Can you work these out from the model? Positions are in its coordinate system, mm. A direction names the side the tool comes from. Give positions to 0.01 mm unless a question says otherwise; leave off trailing zeros. Write each loop counter-clockwise with the first axis right and the second up, starting at its lowest first coordinate (ties: lowest second). Pieces come first, ordered by that corner, then holes.
1. Suppose I cut it at A-A (y = 0). Please give me the cut outline in (x, z).
2. Suppose I cut it at C-C (x = -20.5). Please give me the cut outline in (y, z), and give its area (3 significant figures).
3. On a 3-axis mill with a long thin cutter (end or side, diameter ignored), from which of +Z, -Z, +X, -X, +Y, -Y can I reach the whole of each face in a straight line? I mean faces 1 (the cylindrical face through (-6, 0, 91)), 2 (the flat face through (5, -5, 0)), 3 (the cylindrical face through (5.723, -1.802, 8.536)). Say none if no direction works.
4. I'm going to push flat-ended pins straight in: pin 1 (4 mm diameter, centred on x = -7, z = 67, fed in from +Y); pin 2 (12 mm diameter, centred on x = -18.5, z = 29, fed in from +Y); pin 3 (10 mm diameter, centred on x = -5.5, z = 74, fed in from -Y). Where does each tip first touch, or does it pass through?
5. Suppose I cut it at D-D (z = 70.5). Please give me the cut outline in (x, y), and give its area (3 significant figures).
6. If I drill on probe 1 along Y at (x, z) = (0, 95); probe 2 along Z at (x, y) = (-4.5, 6), over which ranges is the centre line in solid material (lowest first)?
7. Thinking about a two-plate mould opening in X: for faces 4 (the cylindrical face through (-2.11, -0.34, 65.48)), 5 (the cylindrical face through (-0.35, -1.269, 34.667)), 6 (the cylindrical face through (23.09, -9.58, 49.3)), which applies, pulls with the +X half, pulls with the -X half, needs draft (parallel to the pull), parting line crosses it, or undercut?
8. Suppose I cut it at B-B (x = 0). Please give me the cut outline in (y, z), and give its area (3 significant figures).
```python
from build123d import *

# Parameters (mm, degrees)
F0_R          = 25
F1_DEPTH      = 100
F2_R          = 9.75
F3_DEPTH      = 25.001
F3_DEPTH_BACK = 25
F4_R          = 9.75
F5_DEPTH      = 25.0010001
F5_DEPTH_BACK = 25
F6_R          = 6
F7_DEPTH      = 25
F8_R          = 6
F9_DEPTH      = 25


with BuildPart() as f1:
    # F0 (on Top) → F1 (new body)
    with BuildSketch(Plane.XY):
        Circle(F0_R)
    extrude(amount=F1_DEPTH)

    # F2 (on Right) → F3 (cut, two sides)
    with BuildSketch(Plane.YZ) as f3_sk:
        with Locations((0, 25)):
            Circle(F2_R)
    extrude(amount=F3_DEPTH, mode=Mode.SUBTRACT)
    extrude(f3_sk.sketch, amount=-F3_DEPTH_BACK, mode=Mode.SUBTRACT)

    # F4 (on Front) → F5 (cut, two sides)
    with BuildSketch(Plane.XZ) as f5_sk:
        with Locations((0, 75)):
            Circle(F4_R)
    extrude(amount=-F5_DEPTH, mode=Mode.SUBTRACT)
    extrude(f5_sk.sketch, amount=F5_DEPTH_BACK, mode=Mode.SUBTRACT)

    # F6 (on face) → F7 (cut)
    with BuildSketch(Plane.XY.offset(100)):
        Circle(F6_R)
    extrude(amount=-F7_DEPTH, mode=Mode.SUBTRACT)

    # F8 (on face) → F9 (cut)
    with BuildSketch(Plane(origin=(0, 0, 0), x_dir=(1, 0, 0), z_dir=(0, 0, -1))):
        Circle(F8_R)
    extrude(amount=-F9_DEPTH, mode=Mode.SUBTRACT)


solid = f1.part
```
Checks:
1. outline: (-25, 0) - (-6, 0) - (-6, 15.25) - (-25, 15.25) - close; (-25, 34.75) - (25, 34.75) - (25, 100) - (6, 100) - (6, 82.69) arc R9.75 cw (long way) to (-6, 82.69) - (-6, 100) - (-25, 100) - close; (6, 0) - (25, 0) - (25, 15.25) - (6, 15.25) - close
2. outline: (-14.31, 0) - (14.31, 0) - (14.31, 100) - (-14.31, 100) - close; hole circle Ø19.5 at (0, 25)
2. area: 2,560 mm2
3. face 1: +Z
3. face 2: -Z, +X, -X, +Y, -Y
3. face 3: -Z
4. pin 1: stops at y = 24.49
4. pin 2: stops at y = 21.65
4. pin 3: stops at y = -23.59
5. outline: (-8.65, -23.46) - (-8.65, 23.46) arc R25 ccw to start; (8.65, -23.46) arc R25 ccw to (8.65, 23.46) - close
5. area: 1,120 mm2
6. probe 1: y = -25 to -6, 6 to 25
6. probe 2: z = 0 to 17.31, 32.69 to 66.35, 83.65 to 100
7. face 4: undercut
7. face 5: needs draft
7. face 6: parting line crosses it
8. outline: (-25, 0) - (-6, 0) - (-6, 17.31) arc R9.75 cw (long way) to (6, 17.31) - (6, 0) - (25, 0) - (25, 65.25) - (-25, 65.25) - close; (-25, 84.75) - (-6, 84.75) - (-6, 100) - (-25, 100) - close; (6, 84.75) - (25, 84.75) - (25, 100) - (6, 100) - close
8. area: 3,350 mm2
